```python
from build123d import *

# Parameters (mm, degrees)
F0_W     = 90
F0_H     = 45
F1_DEPTH = 5
F0_W_2   = 99.999998
F0_H_2   = 54.999998
F2_DEPTH = 30
F3_W     = 10
F3_H     = 15
F3_H_2   = 5
F4_DEPTH = 5
F5_DEPTH = 20
F6_W     = 10
F6_H     = 5
F7_DEPTH = 10


with BuildPart() as f1:
    # F0 (on Top) → F1 (new body)
    with BuildSketch(Plane.XY):
        with Locations((-45, 22.5)):
            Rectangle(F0_W, F0_H)
    extrude(amount=F1_DEPTH)

    # F0 (on Top) → F2 (join)
    with BuildSketch(Plane.XY):
        with Locations((-45, 22.5)):
            Rectangle(F0_W_2, F0_H_2)
        with Locations((-45, 22.5)):
            Rectangle(F0_W, F0_H, mode=Mode.SUBTRACT)
    extrude(amount=F2_DEPTH)

    # F3 (on face) → F4 (join)
    with BuildSketch(Plane.XY.offset(30)):
        with Locations((-79.999999, 57.499999)):
            Rectangle(F3_W, F3_H)
        with Locations((-79.999999, 67.499999)):
            Rectangle(F3_W, F3_H_2)
        with Locations((-10.000001, 57.499999)):
            Rectangle(F3_W, F3_H)
        with Locations((-10.000001, 67.499999)):
            Rectangle(F3_W, F3_H_2)
    extrude(amount=-F4_DEPTH)

    # F3 (on face) → F5 (join)
    with BuildSketch(Plane.XY.offset(30)):
        with Locations((-79.999999, 67.499999)):
            Rectangle(F3_W, F3_H_2)
        with Locations((-10.000001, 67.499999)):
            Rectangle(F3_W, F3_H_2)
    extrude(amount=-F5_DEPTH)

    # F6 (on face) → F7 (join)
    with BuildSketch(Plane(origin=(0, 49.999999, 0), x_dir=(-1, 0, 0), z_dir=(0, 1, 0))):
        with Locations((10.000001, 12.5)):
            Rectangle(F6_W, F6_H)
        with Locations((79.999999, 12.5)):
            Rectangle(F6_W, F6_H)
    extrude(amount=F7_DEPTH)


solid = f1.part
```
Here's how the part is built. I have some questions about the finished solid (model axes, mm). A direction names the side the tool comes from. Give positions to 0.01 mm unless a question says otherwise; leave off trailing zeros. Loops run counter-clockwise (first coordinate to the right, second up) from the corner with the lowest first, then second, coordinate; pieces in that order, holes last. Notation, with made-up numbers: M 36.25,47 L 56.25,47 A13 cw 56.25,60 Z; hole C -23.5,89 d10. An arc over 180 degrees is marked long. Put each result on its own line as item: value. Start each with the question number.
(1) If we mould it in two halves opening along Y, with no side actions, what happens to faces 1 (the flat face through (-45, 47, 30)), 2 (the flat face through (-46, 45, 17)), 3 (the flat face through (-10, 70, 20))? For each: +Y half, -Y half, draft (parallel to the pull), parting line (faces both ways), or undercut.
(2) I want a section at D-D on z = 26.25. Please give me the cut outline in (x, y).
(3) I want a section at B-B on y = 55. Please give me the cut outline in (x, z).
(4) I want a section at A-A on z = 17. Please give me the cut outline in (x, y), then the cut area to 3 significant figures.
(5) Will these pins go through, and if not, where does the flat tip stop? pin 1 Ø1.5 at (x, y) = (-6, 44) entering from +Z; pin 2 Ø5.5 at (x, y) = (-81.5, 68.5) entering from -Z; pin 3 Ø4 at (y, z) = (55.5, 12) entering from -X.
(6) I need wall thicknesses on line 1 along Y through (x, z) = (-83, 19.5); line 2 along X through (y, z) = (41, 12.5); line 3 along Y through (x, z) = (-43, 13). Which ranges of each line are inside material? Lowest first, please. Write a range as [from, to].
(7) I want a section at C-C on x = -67.5. Please give me the cut outline in (y, z), then the cut area to 3 significant figures.
(8) For faces 4 (the flat face through (-85, 67, 25)), 5 (the flat face through (-80, 55, 10)), 6 (the flat face through (-80, 55, 15)), which set-ups out of +Z, -Z, +X, -X, +Y, -Y let a thin tool reach every point of the face, with its end or its side?
Answer block:
1. face 1: draft
1. face 2: undercut
1. face 3: +Y half
2. outline: M -95,-5 L 5,-5 L 5,50 L -5,50 L -5,70 L -15,70 L -15,50 L -75,50 L -75,70 L -85,70 L -85,50 L -95,50 Z; hole M -90,0 L 0,0 L 0,45 L -90,45 Z
3. outline: M -85,10 L -75,10 L -75,15 L -85,15 Z; M -85,25 L -75,25 L -75,30 L -85,30 Z; M -15,10 L -5,10 L -5,15 L -15,15 Z; M -15,25 L -5,25 L -5,30 L -15,30 Z
4. outline: M -95,-5 L 5,-5 L 5,50 L -95,50 Z; M -85,65 L -75,65 L -75,70 L -85,70 Z; M -15,65 L -5,65 L -5,70 L -15,70 Z; hole M -90,0 L 0,0 L 0,45 L -90,45 Z
4. area: 1,550 mm^2
5. pin 1: z = 5
5. pin 2: z = 10
5. pin 3: x = -85
6. line 1: [-5, 0], [45, 50], [65, 70]
6. line 2: [-95, -90], [0, 5]
6. line 3: [-5, 0], [45, 50]
7. outline: M -5,0 L 50,0 L 50,30 L 45,30 L 45,5 L 0,5 L 0,30 L -5,30 Z
7. area: 525 mm^2
8. face 4: +Z, -Z, -X, +Y
8. face 5: -Z, +X, -X, +Y
8. face 6: +X, -X
